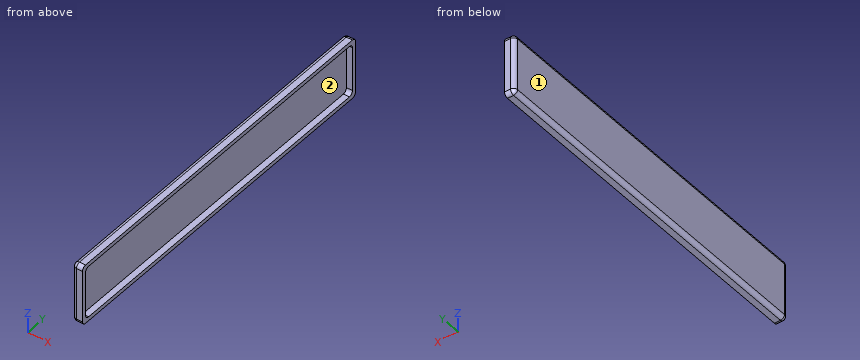
```python
from build123d import *

# Parameters (mm, degrees)
BOX007_W          = 3
BOX007_H          = 176
BOX007_DEPTH      = 26
FILLET003_R       = 2
BOX005_W          = 2
BOX005_H          = 176
BOX005_DEPTH      = 26
CYLINDER021_R     = 2
CYLINDER021_DEPTH = 26
CYLINDER022_R     = 2
CYLINDER022_DEPTH = 26
CYLINDER023_R     = 2
CYLINDER023_DEPTH = 176
CYLINDER024_R     = 2
CYLINDER024_DEPTH = 176
BOX006_W          = 3
BOX006_H          = 180
BOX006_DEPTH      = 30
FILLET002_R       = 2


with BuildPart() as fillet003:
    # Box007 → Box007 (new body)
    with BuildSketch(Plane(origin=(7, 2, 2), x_dir=(1, 0, 0), z_dir=(0, 0, 1))):
        with Locations((1.5, 88)):
            Rectangle(BOX007_W, BOX007_H)
    extrude(amount=BOX007_DEPTH)

    # Fillet003
    fillet003_edges = [fillet003.edges().sort_by_distance(p)[0] for p in [
        (8.5, 2, 2),
        (8.5, 2, 28),
        (8.5, 178, 2),
        (8.5, 178, 28),
    ]]
    fillet(fillet003_edges, radius=FILLET003_R)


with BuildPart() as fillet003_1:
    # Fillet003 placement: moved
    add(fillet003.part.moved(Location((-5, 0, 0))))


with BuildPart() as cube005:
    # Box005 → Box005 (new body)
    with BuildSketch(Plane(origin=(0, 2, 2), x_dir=(1, 0, 0), z_dir=(0, 0, 1))):
        with Locations((1, 88)):
            Rectangle(BOX005_W, BOX005_H)
    extrude(amount=BOX005_DEPTH)


with BuildPart() as cylinder021:
    # Cylinder021 → Cylinder021 (new body)
    with BuildSketch(Plane(origin=(2, 2, 2), x_dir=(0, 1, 0), z_dir=(0, 0, 1))):
        Circle(CYLINDER021_R)
    extrude(amount=CYLINDER021_DEPTH)


with BuildPart() as cylinder022:
    # Cylinder022 → Cylinder022 (new body)
    with BuildSketch(Plane(origin=(2, 178, 2), x_dir=(0, 1, 0), z_dir=(0, 0, 1))):
        Circle(CYLINDER022_R)
    extrude(amount=CYLINDER022_DEPTH)


with BuildPart() as cylinder023:
    # Cylinder023 → Cylinder023 (new body)
    with BuildSketch(Plane(origin=(2, 178, 2), x_dir=(1, 0, 0), z_dir=(0, -1, 0))):
        Circle(CYLINDER023_R)
    extrude(amount=CYLINDER023_DEPTH)


with BuildPart() as cylinder024:
    # Cylinder024 → Cylinder024 (new body)
    with BuildSketch(Plane(origin=(2, 178, 28), x_dir=(1, 0, 0), z_dir=(0, -1, 0))):
        Circle(CYLINDER024_R)
    extrude(amount=CYLINDER024_DEPTH)


with BuildPart() as sphere005:
    # Sphere004 → Sphere004 (revolve)
    with BuildSketch(Plane(origin=(2, 2, 2), x_dir=(1, 0, 0), z_dir=(0, -1, 0))):
        with BuildLine():
            ThreePointArc((0, -2), (2, 0), (0, 2))
            Line((0, 2), (0, -2))
        make_face()
    revolve(axis=Axis((2, 2, 2), (0, 0, 1)))


with BuildPart() as sphere006:
    # Sphere005 → Sphere005 (revolve)
    with BuildSketch(Plane(origin=(2, 178, 2), x_dir=(1, 0, 0), z_dir=(0, -1, 0))):
        with BuildLine():
            ThreePointArc((0, -2), (2, 0), (0, 2))
            Line((0, 2), (0, -2))
        make_face()
    revolve(axis=Axis((2, 178, 2), (0, 0, 1)))


with BuildPart() as sphere007:
    # Sphere006 → Sphere006 (revolve)
    with BuildSketch(Plane(origin=(2, 2, 28), x_dir=(1, 0, 0), z_dir=(0, -1, 0))):
        with BuildLine():
            ThreePointArc((0, -2), (2, 0), (0, 2))
            Line((0, 2), (0, -2))
        make_face()
    revolve(axis=Axis((2, 2, 28), (0, 0, 1)))


with BuildPart() as sphere008:
    # Sphere007 → Sphere007 (revolve)
    with BuildSketch(Plane(origin=(2, 178, 28), x_dir=(1, 0, 0), z_dir=(0, -1, 0))):
        with BuildLine():
            ThreePointArc((0, -2), (2, 0), (0, 2))
            Line((0, 2), (0, -2))
        make_face()
    revolve(axis=Axis((2, 178, 28), (0, 0, 1)))


with BuildPart() as cut027:
    # Box006 → Box006 (new body)
    with BuildSketch(Plane(origin=(2, 0, 0), x_dir=(1, 0, 0), z_dir=(0, 0, 1))):
        with Locations((1.5, 90)):
            Rectangle(BOX006_W, BOX006_H)
    extrude(amount=BOX006_DEPTH)

    # Fillet002
    fillet002_edges = [cut027.edges().sort_by_distance(p)[0] for p in [
        (3.5, 0, 0),
        (3.5, 0, 30),
        (3.5, 180, 0),
        (3.5, 180, 30),
    ]]
    fillet(fillet002_edges, radius=FILLET002_R)

    # Fusion001: union Cube005, Cylinder021, Cylinder022, Cylinder023, Cylinder024, Sphere005, Sphere006, Sphere007, Sphere008
    add(cube005.part)
    add(cylinder021.part)
    add(cylinder022.part)
    add(cylinder023.part)
    add(cylinder024.part)
    add(sphere005.part)
    add(sphere006.part)
    add(sphere007.part)
    add(sphere008.part)

    # Cut027: cut Fillet003
    add(fillet003_1.part, mode=Mode.SUBTRACT)


solid = cut027.part
```
Could you check a few things on this model? Use its own coordinates, in mm. Face numbers are marked on the shaded views. Coordinates: 2 decimals unless noted, no trailing zeros. Loops run counter-clockwise (first coordinate to the right, second up) from the corner with the lowest first, then second, coordinate; pieces in that order, holes last. Notation, with made-up numbers: M 45,26 L 72,26 A16 cw 72,54 Z; hole C -23.75,31.25 d8. An arc over 180 degrees is marked long. Put each result on its own line as item: value. Start each with the question number.
(1) Suppose I cut it at A-A on x = 3.9. Please give me the cut outline in (y, z).
(2) I need wall thicknesses on line 1 (Y direction, x = 4.7, z = 10); line 2 (Z direction, x = 2.3, y = 85); line 3 (Z direction, x = 1.7, y = 148.5). Which ranges of each line are inside material? Lowest first, please. Write a range as from..to.
(3) Will these pins go through, and if not, where does the flat tip stop? P1, Ø5, axis at y = 103.5, z = 18.5, coming from the +X side; P2, Ø4, axis at y = 78, z = 16.5, coming from the -X side; P3, Ø1.5, axis at x = 1, z = 23, coming from the -Y side.
(4) Suppose I cut it at B-B on z = 18. Please give me the cut outline in (x, y), then the cut area to 3 significant figures.
(5) Suppose I cut it at C-C on y = 155.5. Please give me the cut outline in (x, z).
(6) Thinking about a two-plate mould opening in Y: for the marked faces 1 and 2, which applies, pulls with the +Y half, pulls with the -Y half, needs draft (parallel to the pull), parting line crosses it, or undercut?
Solutions:
1. outline: M 0,2 A2 ccw 2,0 L 178,0 A2 ccw 180,2 L 180,28 A2 ccw 178,30 L 2,30 A2 ccw 0,28 Z; hole M 2,4 A2 ccw 4,2 L 176,2 A2 ccw 178,4 L 178,26 A2 ccw 176,28 L 4,28 A2 ccw 2,26 Z
2. line 1: y = 0..2, 178..180
2. line 2: z = 0..2, 28..30
2. line 3: z = 0.02..29.98
3. P1: stops at x = 2
3. P2: stops at x = 0
3. P3: stops at y = 0.02
4. outline: M 0,2 A2 ccw 2,0 L 5,0 L 5,2 L 2,2 L 2,178 L 5,178 L 5,180 L 2,180 A2 ccw 0,178 Z
4. area: 370 mm2
5. outline: M 0,2 A2 ccw 2,0 L 5,0 L 5,2 L 2,2 L 2,28 L 5,28 L 5,30 L 2,30 A2 ccw 0,28 Z
6. face 1: needs draft
6. face 2: undercut
